```python
from build123d import *

# Parameters (mm, degrees)
F0_W     = 460.375
F0_H     = 609.6
F1_DEPTH = 914.4
F2_T     = -12.7
F3_W     = 460.375
F3_H     = 914.4
F3_W_2   = 444.5
F3_H_2   = 901.7
F3_W_3   = 434.975
F3_H_3   = 889
F3_W_4   = 377.825
F3_H_4   = 831.85
F4_DEPTH = 19.05
F3_W_5   = 330.2
F3_H_5   = 787.4
F5_DEPTH = 19.05
F6_W     = 330.2
F6_H     = 7.9375
F7_DEPTH = 787.4
F8_SIZE  = 3.175


with BuildPart() as f1:
    # F0 (on Top) → F1 (new body)
    with BuildSketch(Plane.XY):
        Rectangle(F0_W, F0_H)
    extrude(amount=F1_DEPTH)

    # F2
    f2_openings = [f1.faces().sort_by_distance(p)[0] for p in [
        (0, -304.8, 457.2),
    ]]
    offset(amount=F2_T, openings=f2_openings)

    # F3 (on face) → F4 (join)
    with BuildSketch(Plane.XZ.offset(304.8)):
        with Locations((0, 457.2)):
            Rectangle(F3_W, F3_H)
        with Locations((0, 457.2)):
            Rectangle(F3_W_2, F3_H_2, mode=Mode.SUBTRACT)
        with Locations((0, 457.2)):
            Rectangle(F3_W_3, F3_H_3)
        with Locations((0, 457.2)):
            Rectangle(F3_W_4, F3_H_4, mode=Mode.SUBTRACT)
    extrude(amount=-F4_DEPTH)

    # F3 (on face) → F5 (join)
    with BuildSketch(Plane.XZ.offset(304.8)):
        with Locations((0, 457.2)):
            Rectangle(F3_W_3, F3_H_3)
        with Locations((0, 457.2)):
            Rectangle(F3_W_4, F3_H_4, mode=Mode.SUBTRACT)
        with Locations((0, 457.2)):
            Rectangle(F3_W_4, F3_H_4)
        with Locations((0, 457.2)):
            Rectangle(F3_W_5, F3_H_5, mode=Mode.SUBTRACT)
    extrude(amount=F5_DEPTH)

    # F6 (on face) → F7 (join, through all)
    with BuildSketch(Plane(origin=(0, 0, 850.9), x_dir=(1, 0, 0), z_dir=(0, 0, -1))):
        with Locations((0, 313.53125)):
            Rectangle(F6_W, F6_H)
    extrude(amount=F7_DEPTH)

    # F8
    f8_edges = [f1.edges().sort_by_distance(p)[0] for p in [
        (0, -323.85, 63.5),
        (-165.1, -323.85, 457.2),
        (165.1, -323.85, 457.2),
        (0, -323.85, 850.9),
        (-230.1875, 304.8, 457.2),
    ]]
    chamfer(f8_edges, length=F8_SIZE)


solid = f1.part
```
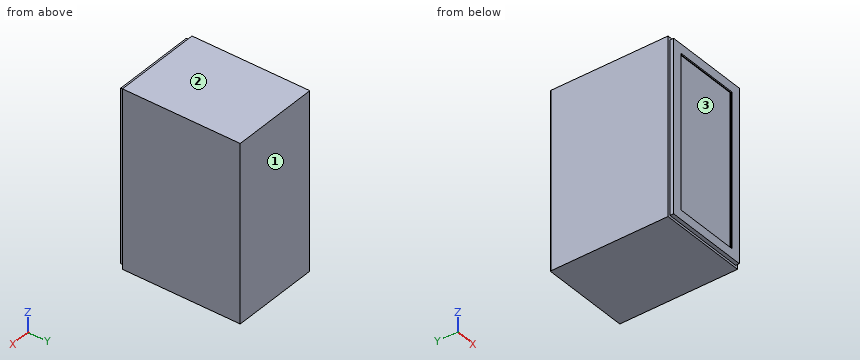
For this review, take the finished solid that the model builds, in its own axes (mm). Face numbers are marked on the shaded views. Coordinates: 2 decimals unless noted, no trailing zeros. Write each loop counter-clockwise with the first axis right and the second up, starting at its lowest first coordinate (ties: lowest second). Pieces come first, ordered by that corner, then holes. Notation, with made-up numbers: (73.25, -26.75) - (82.25, -26.75) arc R19 cw to (82.25, 6.25) - close; hole circle Ø5 at (2.5, 75.5). An arc over 180 degrees is marked (long way). Put each result on its own line as item: value.
1. Wall thickness on probe 1 along Z at (x, y) = (-70.5, -175); probe 2 along X at (y, z) = (-94.5, 354); probe 3 along Y at (x, z) = (-172.5, 871): over which ranges is each line inside the solid? List them lowest first.
Values found:
probe 1: 0 to 12.7, 901.7 to 914.4
probe 2: -230.19 to -217.49, 217.49 to 230.19
probe 3: -323.85 to -304.8, 292.1 to 304.8
2. Add section C-C, the plane y = -161. Give the boundary of the cut face in (x, z), then the cut area to 3 significant figures.
Values found:
outline: (-230.19, 0) - (230.19, 0) - (230.19, 914.4) - (-230.19, 914.4) - close; hole (-217.49, 12.7) - (217.49, 12.7) - (217.49, 901.7) - (-217.49, 901.7) - close
area: 34,300 mm²
3. For pin 1 (3.5 mm diameter, centred on y = -319.5, z = 519, fed in from +X); pin 2 (9.5 mm diameter, centred on x = -58, y = -315, fed in from +Z); pin 3 (3.5 mm diameter, centred on x = 80.5, y = -318.5, fed in from -Z), all flat-tipped, find the tip position at first contact; note any pin that passes through.
Values found:
pin 1: x = 217.49
pin 2: z = 901.7
pin 3: z = 12.7
4. Mouldability with a two-part tool opening along Z and no side actions: class the marked faces 1, 2 and 3 as released by +Z, released by -Z, zero draft, split by the parting line, or undercut.
Values found:
face 1: zero draft
face 2: released by +Z
face 3: undercut
